Work out the finished part from the listing and answer in its coordinate system (mm). A direction names the side the tool comes from. Give positions to 0.01 mm unless a question says otherwise; leave off trailing zeros. Loops run counter-clockwise (first coordinate to the right, second up) from the corner with the lowest first, then second, coordinate; pieces in that order, holes last. Notation, with made-up numbers: M 6.5,13 L 33.5,13 A15 cw 33.5,18 Z; hole C -18.5,3 d1. An arc over 180 degrees is marked long. Use a Markdown table: item, result.
```python
from build123d import *

# Parameters (mm, degrees)
SKETCH1_R           = 4.191
BOSS_EXTRUDE1_DEPTH = 1.1811
SKETCH2_R           = 0.8001
BOSS_EXTRUDE2_DEPTH = 25.4
FILLET1_R           = 0.508


with BuildPart() as part:
    # Sketch1 → Boss-Extrude1 (new, symmetric)
    with BuildSketch(Plane.XY):
        Circle(SKETCH1_R)
    extrude(amount=BOSS_EXTRUDE1_DEPTH, both=True)

    # Sketch2 → Boss-Extrude2 (add)
    with BuildSketch(Plane(origin=(0, 0, 0), x_dir=(1, 0, 0), z_dir=(0, 1, 0))):
        with Locations(Location((0, 0, 0), (0, 0, 90))):
            Circle(SKETCH2_R)
    extrude(amount=BOSS_EXTRUDE2_DEPTH)

    # Fillet1
    fillet1_edges = [part.edges().sort_by_distance(p)[0] for p in [
        (0, 4.191, 0.8001),
    ]]
    fillet(fillet1_edges, radius=FILLET1_R)


solid = part.part
```
(1) A cutting plane is placed at B-B (x = -1.75). Write down the section's boundary in (y, z).
Entries:
| item | result |
|---|---|
| outline | M -3.81,-1.18 L 3.81,-1.18 L 3.81,1.18 L -3.81,1.18 Z |
(2) A cutting plane is placed at C-C (x = 3.25). Write down the section's boundary in (y, z).
Entries:
| item | result |
|---|---|
| outline | M -2.65,-1.18 L 2.65,-1.18 L 2.65,1.18 L -2.65,1.18 Z |
(3) Consider probe 1 along X at (y, z) = (19.75, 0.05); probe 2 along X at (y, z) = (12.5, 0.35); probe 3 along Y at (x, z) = (0.75, 0.8). Determine where each line is inside the solid, lowest interval first. Write a range as [from, to].
Entries:
| item | result |
|---|---|
| probe 1 | x = [-0.8, 0.8] |
| probe 2 | x = [-0.72, 0.72] |
| probe 3 | y = [-4.12, 4.15] |
(4) Which of the six approach directions +Z, -Z, +X, -X, +Y, -Y give full straight-line access (tool end or side, diameter ignored) to faces 1 (the flat face through (0, 0, 1.181)), 2 (the cylindrical face through (0.78, 14.81, 0.17))?
Entries:
| item | result |
|---|---|
| face 1 | +Z, +X, -X, +Y, -Y |
| face 2 | +Y |
(5) A cutting plane is placed at A-A (y = 7.25). Write down the section's boundary in (x, z), and give its area (3 significant figures).
Entries:
| item | result |
|---|---|
| outline | C 0,0 d1.6 |
| area | 2.01 mm² |
